```python
from build123d import *

# Parameters (mm, degrees)
BOSS_EXTRUDE1_DEPTH      = 45
BOSS_EXTRUDE1_DEPTH_BACK = 45
BOSS_EXTRUDE2_DEPTH      = 22.5


with BuildPart() as part:
    # Sketch1 → Boss-Extrude1 (new, two sides: drawn at the far end of the back side and taken through both)
    with BuildSketch(Plane.XY.offset(-BOSS_EXTRUDE1_DEPTH_BACK)):
        with BuildLine():
            Line((-67.5, 0), (67.5, 0))
            Line((67.5, 0), (67.5, 45))
            Line((67.5, 45), (45, 45))
            Line((45, 45), (45, 100))
            ThreePointArc((45, 100), (0, 145), (-45, 100))
            Line((-45, 100), (-45, 45))
            Line((-45, 45), (-67.5, 45))
            Line((-67.5, 45), (-67.5, 0))
        make_face()
        with BuildLine():
            Line((-35, 35), (-35, 100))
            ThreePointArc((-35, 100), (0, 135), (35, 100))
            Line((35, 100), (35, 35))
            Line((35, 35), (57.5, 35))
            Line((57.5, 35), (57.5, 10))
            Line((57.5, 10), (-57.5, 10))
            Line((-57.5, 10), (-57.5, 35))
            Line((-57.5, 35), (-35, 35))
        make_face(mode=Mode.SUBTRACT)
    extrude(amount=BOSS_EXTRUDE1_DEPTH + BOSS_EXTRUDE1_DEPTH_BACK)

    # Sketch2 → Boss-Extrude2 (add)
    with BuildSketch(Plane(origin=(45, 0, 0), x_dir=(0, 0, -1), z_dir=(1, 0, 0))):
        with BuildLine():
            Line((17.5, 65), (17.5, 45))
            Line((17.5, 45), (-17.5, 45))
            Line((-17.5, 45), (-17.5, 65))
            ThreePointArc((-17.5, 65), (0, 82.5), (17.5, 65))
        make_face()
    extrude(amount=BOSS_EXTRUDE2_DEPTH)


solid = part.part
```
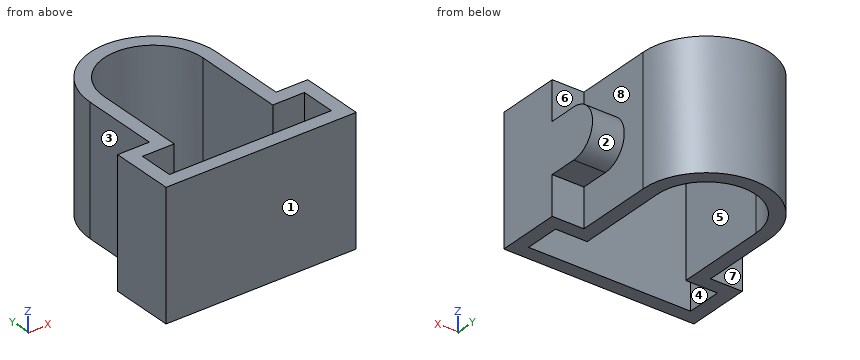
The listing builds one solid part. Answer for the finished solid, in the listing's coordinates (mm). Face numbers are marked on the shaded views. A direction names the side the tool comes from. Give positions to 0.01 mm unless a question says otherwise; leave off trailing zeros. Write each loop counter-clockwise with the first axis right and the second up, starting at its lowest first coordinate (ties: lowest second). Pieces come first, ordered by that corner, then holes. Notation, with made-up numbers: M 87.25,72.25 L 127.25,72.25 A29 cw 127.25,94.25 Z; hole C 24,32.5 d8. An arc over 180 degrees is marked long. Write each question's results on one line, items separated by ' | '.
Q1. For a pull along Y with two mould halves and no side action, classify the marked faces 1, 2, 3 and 4 as released by +Y, released by -Y, zero draft, split by the parting line, or undercut.
Output values:
face 1: released by -Y | face 2: released by +Y | face 3: zero draft | face 4: undercut
Q2. A tool of negligible diameter and unlimited length cuts with its end or side. For the marked faces 5, 6, 7 and 8, from which of +Z, -Z, +X, -X, +Y, -Y can it reach the whole face along a straight path? Write none if from no direction.
Output values:
face 5: +Z, -Z | face 6: +Z, +X, +Y | face 7: +Z, -Z, -X, +Y | face 8: +X, +Y
Q3. Flat-ended cylindrical pins translate along their axes: P1, Ø16, axis at x = 57, y = 59.5, coming from the +Z side; P2, Ø12, axis at y = 127, z = -3.5, coming from the -X side; P3, Ø25, axis at x = 59, z = -36.5, coming from the +Y side; P4, Ø3, axis at x = -32, y = 69.5, coming from the +Z side. Find the tip coordinate at first contact, or state that the pin passes through.
Output values:
P1: z = 17.5 | P2: x = -39.8 | P3: y = 45 | P4: through
Q4. Section D-D, the plane y = 20.5 is taken. Write down the section's boundary in (x, z), then the cut area to 3 significant figures.
Output values:
outline: M -67.5,-45 L -57.5,-45 L -57.5,45 L -67.5,45 Z; M 57.5,-45 L 67.5,-45 L 67.5,45 L 57.5,45 Z | area: 1,800 mm2
Q5. Section B-B, the plane x = 50 is taken. Write down the section's boundary in (y, z), then the cut area to 3 significant figures.
Output values:
outline: M 0,-45 L 10,-45 L 10,45 L 0,45 Z; M 35,-45 L 45,-45 L 45,-17.5 L 65,-17.5 A17.5 ccw 65,17.5 L 45,17.5 L 45,45 L 35,45 Z | area: 2,980 mm2
Q6. Section C-C, the plane z = 0 is taken. Write down the section's boundary in (x, y), then the cut area to 3 significant figures.
Output values:
outline: M -67.5,0 L 67.5,0 L 67.5,82.5 L 45,82.5 L 45,100 A45 ccw -45,100 L -45,45 L -67.5,45 Z; hole M -57.5,10 L 57.5,10 L 57.5,35 L 35,35 L 35,100 A35 ccw -35,100 L -35,35 L -57.5,35 Z | area: 5,700 mm2
Q7. Consider L1, parallel to X at y = 10.5, z = 27; L2, parallel to X at y = 73, z = -1; L3, parallel to Y at x = 49.5, z = 20. Determine where each line is inside the solid, lowest interval first. Write a range as from..to.
Output values:
L1: -67.5..-57.5, 57.5..67.5 | L2: -45..-35, 35..67.5 | L3: 0..10, 35..45
Q8. Section A-A, the plane y = 59 is taken. Write down the section's boundary in (x, z).
Output values:
outline: M -45,-45 L -35,-45 L -35,45 L -45,45 Z; M 35,-45 L 45,-45 L 45,-17.5 L 67.5,-17.5 L 67.5,17.5 L 45,17.5 L 45,45 L 35,45 Z
